Design review of the part built by this model. Coordinates are the model's own, in mm. Round coordinates to 2 decimals unless told otherwise and drop trailing zeros. Loops run counter-clockwise (first coordinate to the right, second up) from the corner with the lowest first, then second, coordinate; pieces in that order, holes last. Notation, with made-up numbers: (22.25, 39.25) -> (36.25, 39.25) arc R16 ccw to (36.25, 48.25) -> close; hole circle Ø1 at (-5.75, 46). An arc over 180 degrees is marked (long way). Write each question's results on one line, items separated by ' | '. Start each with the question number.
from build123d import *

# Parameters (mm, degrees)
SKETCH1_W           = 279.4
SKETCH1_H           = 279.4
BOSS_EXTRUDE1_DEPTH = 5.08
FILLET1_R           = 25.4
SKETCH2_W           = 5.08
SKETCH2_H           = 31.75
CUT_EXTRUDE1_DEPTH  = 396.163923455
SKETCH3_W           = 5.08
SKETCH3_H           = 58.166
CUT_EXTRUDE2_DEPTH  = 396.163923455
SKETCH5_R           = 1.905
CUT_EXTRUDE4_DEPTH  = 396.163923455
CUT_EXTRUDE6_DEPTH  = 396.163923455


with BuildPart() as part:
    # Sketch1 → Boss-Extrude1 (new body)
    with BuildSketch(Plane(origin=(0, 0, 0), x_dir=(1, 0, 0), z_dir=(0, 1, 0))):
        with Locations((139.7, 139.7)):
            Rectangle(SKETCH1_W, SKETCH1_H)
    extrude(amount=BOSS_EXTRUDE1_DEPTH)

    # Fillet1
    fillet1_edges = [part.edges().sort_by_distance(p)[0] for p in [
        (0, 2.54, -279.4),
        (279.4, 2.54, -279.4),
        (279.4, 2.54, 0),
        (0, 2.54, 0),
    ]]
    fillet(fillet1_edges, radius=FILLET1_R)

    # Sketch2 → Cut-Extrude1 (cut, through all)
    with BuildSketch(Plane(origin=(0, 5.08, 0), x_dir=(1, 0, 0), z_dir=(0, 1, 0))):
        with Locations((66.04, 243.205)):
            Rectangle(SKETCH2_W, SKETCH2_H)
        with Locations((213.36, 243.205)):
            Rectangle(SKETCH2_W, SKETCH2_H)
        with Locations((66.04, 36.195)):
            Rectangle(SKETCH2_W, SKETCH2_H)
        with Locations((213.36, 36.195)):
            Rectangle(SKETCH2_W, SKETCH2_H)
    extrude(amount=-CUT_EXTRUDE1_DEPTH, mode=Mode.SUBTRACT)

    # Sketch3 → Cut-Extrude2 (cut, through all)
    with BuildSketch(Plane(origin=(0, 5.08, 0), x_dir=(1, 0, 0), z_dir=(0, 1, 0))):
        with Locations((8.89, 139.7)):
            Rectangle(SKETCH3_W, SKETCH3_H)
        with Locations((270.51, 139.7)):
            Rectangle(SKETCH3_W, SKETCH3_H)
        with Locations((39.37, 139.7)):
            Rectangle(SKETCH3_W, SKETCH3_H)
        with Locations((240.03, 139.7)):
            Rectangle(SKETCH3_W, SKETCH3_H)
    extrude(amount=-CUT_EXTRUDE2_DEPTH, mode=Mode.SUBTRACT)

    # Sketch5 → Cut-Extrude4 (cut, through all)
    with BuildSketch(Plane.XZ):
        with Locations(Location((115.062, -12.7, 0), (0, 0, 270))):
            Circle(SKETCH5_R)
        with Locations(Location((164.338, -12.7, 0), (0, 0, 270))):
            Circle(SKETCH5_R)
        with Locations(Location((164.338, -51.308, 0), (0, 0, 270))):
            Circle(SKETCH5_R)
        with Locations(Location((115.062, -51.308, 0), (0, 0, 270))):
            Circle(SKETCH5_R)
    extrude(amount=-CUT_EXTRUDE4_DEPTH, mode=Mode.SUBTRACT)

    # Sketch6 → Cut-Extrude6 (cut, through all)
    with BuildSketch(Plane(origin=(0, 5.08, 0), x_dir=(1, 0, 0), z_dir=(0, 1, 0))):
        Polygon((117.82964184, 192.499715283), (118.801657759, 190.15306127), (139.7, 194.31), (139.7, 196.85), align=None)
        Polygon((82.55, 139.7), (86.900284717, 117.82964184), (89.24693873, 118.801657759), (85.09, 139.7), align=None)
        Polygon((160.598342241, 89.24693873), (161.57035816, 86.900284717), (139.7, 82.55), (139.7, 85.09), align=None)
        Polygon((196.85, 139.7), (192.499715283, 161.57035816), (190.15306127, 160.598342241), (194.31, 139.7), align=None)
    extrude(amount=-CUT_EXTRUDE6_DEPTH, mode=Mode.SUBTRACT)


solid = part.part
1) To check wall thickness, follow line 1 (X direction, y = 1.5, z = -49); line 2 (Z direction, x = 212, y = 0.65); line 3 (X direction, y = 4, z = -13). State the ranges of each line that lie inside material, in increasing order. Write a range as from..to.
2) Insertion check: pin 1 (3 mm diameter, centred on x = 164.338, z = -12.7, fed in from +Y). The pin has a flat end and moves straight along its axis. Give the tip position at first contact, or say it passes through.
3) Take a section at A-A (z = -39). Write out the cut boundary in (x, y).
4) Take a section at C-C (y = 3.75). State how many separate pieces and enclosed holes the cut face has, plus the area to 3 significant figures.
5) Take a section at B-B (z = -133). Write out the cut boundary in (x, y), plus the area to 3 significant figures.
Geometry check:
1) line 1: x = 0..63.5, 68.58..210.82, 215.9..279.4 | line 2: z = -279.4..-259.08, -227.33..-52.07, -20.32..0 | line 3: x = 3.23..113.18, 116.94..162.46, 166.22..276.17
2) pin 1: passes through
3) outline: (0, 0) -> (63.5, 0) -> (63.5, 5.08) -> (0, 5.08) -> close; (68.58, 0) -> (210.82, 0) -> (210.82, 5.08) -> (68.58, 5.08) -> close; (215.9, 0) -> (279.4, 0) -> (279.4, 5.08) -> (215.9, 5.08) -> close
4) separate pieces: 1 | enclosed holes: 16 | area: 75,400 mm^2
5) outline: (0, 0) -> (6.35, 0) -> (6.35, 5.08) -> (0, 5.08) -> close; (11.43, 0) -> (36.83, 0) -> (36.83, 5.08) -> (11.43, 5.08) -> close; (41.91, 0) -> (83.88, 0) -> (83.88, 5.08) -> (41.91, 5.08) -> close; (86.42, 0) -> (237.49, 0) -> (237.49, 5.08) -> (86.42, 5.08) -> close; (242.57, 0) -> (267.97, 0) -> (267.97, 5.08) -> (242.57, 5.08) -> close; (273.05, 0) -> (279.4, 0) -> (279.4, 5.08) -> (273.05, 5.08) -> close | area: 1,300 mm^2
